Model file for the job. Use its own axes, mm. A direction names the side the tool comes from. Round coordinates to 2 decimals unless told otherwise and drop trailing zeros. Loops run counter-clockwise (first coordinate to the right, second up) from the corner with the lowest first, then second, coordinate; pieces in that order, holes last. Notation, with made-up numbers: (-7, 15) -> (52, 15) arc R37 ccw to (52, 53) -> close; hole circle Ø9 at (88.5, 22). An arc over 180 degrees is marked (long way). Use a Markdown table: item, result.
from build123d import *

# Parameters (mm, degrees)
F0_W      = 110
F0_H      = 110
F1_DEPTH  = 15
F2_W      = 85
F2_H      = 85
F3_DEPTH  = 51
F4_SIZE   = 4
F5_R      = 20
F6_DEPTH  = 66.001
F7_R      = 4.25
F8_DEPTH  = 66.001
F9_R      = 28
F10_DEPTH = 2
F11_R     = 3.25
F12_DEPTH = 25


with BuildPart() as f1:
    # F0 (on Top) → F1 (new body)
    with BuildSketch(Plane.XY):
        with Locations((55, 55)):
            Rectangle(F0_W, F0_H)
    extrude(amount=F1_DEPTH)

    # F2 (on face) → F3 (join)
    with BuildSketch(Plane.XY.offset(15)):
        with Locations((55, 55)):
            Rectangle(F2_W, F2_H)
    extrude(amount=F3_DEPTH)

    # F4
    f4_edges = [f1.edges().sort_by_distance(p)[0] for p in [
        (12.5, 12.5, 40.5),
        (97.5, 12.5, 40.5),
        (97.5, 97.5, 40.5),
        (12.5, 97.5, 40.5),
    ]]
    chamfer(f4_edges, length=F4_SIZE)

    # F5 (on face) → F6 (cut, through all)
    with BuildSketch(Plane.XY.offset(66)):
        with Locations((55, 55)):
            Circle(F5_R)
    extrude(amount=-F6_DEPTH, mode=Mode.SUBTRACT)

    # F7 (on face) → F8 (cut, through all)
    with BuildSketch(Plane(origin=(0, 0, 0), x_dir=(1, 0, 0), z_dir=(0, 0, -1))):
        with Locations((10.5, -10.5)):
            Circle(F7_R)
        with Locations((99.5, -10.5)):
            Circle(F7_R)
        with Locations((99.5, -99.5)):
            Circle(F7_R)
        with Locations((10.5, -99.5)):
            Circle(F7_R)
    extrude(amount=-F8_DEPTH, mode=Mode.SUBTRACT)

    # F9 (on face) → F10 (cut)
    with BuildSketch(Plane(origin=(0, 0, 0), x_dir=(1, 0, 0), z_dir=(0, 0, -1))):
        with Locations((55, -55)):
            Circle(F9_R)
    extrude(amount=-F10_DEPTH, mode=Mode.SUBTRACT)

    # F11 (on face) → F12 (cut)
    with BuildSketch(Plane.XY.offset(66)):
        with BuildLine():
            ThreePointArc((34.317127, 75.682873), (35.021638, 76.737249), (35.26903, 77.98097))
            ThreePointArc((35.26903, 77.98097), (29.016421, 79.224692), (34.317127, 75.682873))
        make_face()
        with Locations((77.98097, 77.98097)):
            Circle(F11_R)
        with Locations((77.98097, 32.01903)):
            Circle(F11_R)
        with Locations((32.01903, 32.01903)):
            Circle(F11_R)
    extrude(amount=-F12_DEPTH, mode=Mode.SUBTRACT)


solid = f1.part
Q1. Band-saw the part on A-A, the plane y = 55. Give the cut face in (x, z), plus the area to 3 significant figures.
Results list:
| item | result |
|---|---|
| outline | (0, 0) -> (27, 0) -> (27, 2) -> (35, 2) -> (35, 66) -> (12.5, 66) -> (12.5, 15) -> (0, 15) -> close; (75, 2) -> (83, 2) -> (83, 0) -> (110, 0) -> (110, 15) -> (97.5, 15) -> (97.5, 66) -> (75, 66) -> close |
| area | 3,310 mm² |
Q2. Pull direction X, two halves, no side cores. Call faces 5 (the face through (103, 56, 15)), 6 (the face through (75.59, 34.22, 53.68)), 7 (the face through (12.5, 54, 40)): released by +X, released by -X, zero draft, split by the parting line, or undercut.
Results list:
| item | result |
|---|---|
| face 5 | zero draft |
| face 6 | undercut |
| face 7 | released by -X |
Q3. Band-saw the part on D-D, the plane x = 99.5. Give the cut face in (y, z).
Results list:
| item | result |
|---|---|
| outline | (0, 0) -> (6.25, 0) -> (6.25, 15) -> (0, 15) -> close; (14.75, 0) -> (95.25, 0) -> (95.25, 15) -> (14.75, 15) -> close; (103.75, 0) -> (110, 0) -> (110, 15) -> (103.75, 15) -> close |
Q4. Flat gauge pins, fed straight in: pin 1 (15.5 mm diameter, centred on y = 38.5, z = 44, fed in from +X); pin 2 (5 mm diameter, centred on x = 77.98, y = 32.02, fed in from +Z); pin 3 (12 mm diameter, centred on y = 30.5, z = 13, fed in from -X); pin 4 (5 mm diameter, centred on x = 99.5, y = 99.5, fed in from -Z). Where does each tip first touch, or does it go through?
Results list:
| item | result |
|---|---|
| pin 1 | stops at x = 97.5 |
| pin 2 | stops at z = 41 |
| pin 3 | stops at x = 0 |
| pin 4 | passes through |
Q5. Band-saw the part on C-C, the plane z = 36. Give the cut face in (x, y).
Results list:
| item | result |
|---|---|
| outline | (12.5, 16.5) -> (16.5, 12.5) -> (93.5, 12.5) -> (97.5, 16.5) -> (97.5, 93.5) -> (93.5, 97.5) -> (16.5, 97.5) -> (12.5, 93.5) -> close; hole circle Ø40 at (55, 55) |
Q6. Drill centre lines: L1, parallel to X at y = 10, z = 10; L2, parallel to Y at x = 99.5, z = 12; L3, parallel to Y at x = 53.5, z = 39. Where is each one in solid material? Low to high. Write a range as from..to.
Results list:
| item | result |
|---|---|
| L1 | x = 0..6.28, 14.72..95.28, 103.72..110 |
| L2 | y = 0..6.25, 14.75..95.25, 103.75..110 |
| L3 | y = 12.5..35.06, 74.94..97.5 |
Q7. Tool access for faces 1 (the face through (78, 78, 41)), 2 (the face through (95, 96, 40)), 3 (the face through (36, 48, 2)), 4 (the face through (14, 15, 40)): list every direction of +Z, -Z, +X, -X, +Y, -Y with a clear straight run to the whole face (end or side of a thin tool).
Results list:
| item | result |
|---|---|
| face 1 | +Z |
| face 2 | +Z, +X, +Y |
| face 3 | -Z |
| face 4 | +Z, -X, -Y |
